from build123d import *


with BuildPart() as part:
    # Sweep1: sweep along a path in Sketch2
    with BuildLine(Plane(origin=(0, 0, 0), x_dir=(1, 0, 0), z_dir=(0, 1, 0))) as sweep1_path:
        Line((-1005, -399), (1005, -399))
        Line((1005, -399), (1005, 399))
        Line((1005, 399), (-1005, 399))
        Line((-1005, 399), (-1005, -399))
    # Sketch3 → Sweep1 (sweep)
    with BuildSketch(Plane.XY):
        Polygon((-955, 0), (-1005, 0), (-1005, 50), (-1000, 50), (-1000, 5), (-955, 5), align=None)
    sweep(path=sweep1_path.line, transition=Transition.RIGHT)


solid = part.part
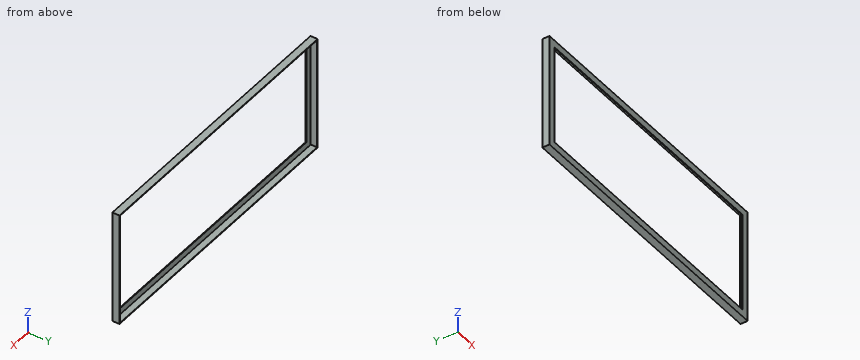
Design review of the part built by this model. Coordinates are the model's own, in mm. Coordinates: 2 decimals unless noted, no trailing zeros. Loops run counter-clockwise (first coordinate to the right, second up) from the corner with the lowest first, then second, coordinate; pieces in that order, holes last. Notation, with made-up numbers: M 12.5,38 L 48.5,38 A23 cw 48.5,72 Z; hole C 73,20 d4. An arc over 180 degrees is marked long. Use one line per item in the form item = value.
(1) Consider section C-C (y = 25). Write out the cut boundary in (x, z).
Return value:
outline = M -1005,-399 L 1005,-399 L 1005,399 L -1005,399 Z; hole M -1000,-394 L 1000,-394 L 1000,394 L -1000,394 Z
(2) Consider section A-A (x = -374). Write out the cut boundary in (y, z), and give its area (3 significant figures).
Return value:
outline = M 0,-399 L 50,-399 L 50,-394 L 5,-394 L 5,-349 L 0,-349 Z; M 0,349 L 5,349 L 5,394 L 50,394 L 50,399 L 0,399 Z
area = 950 mm2
(3) Consider section B-B (z = 168.5). Write out the cut boundary in (x, y), and give its area (3 significant figures).
Return value:
outline = M -1005,0 L -955,0 L -955,5 L -1000,5 L -1000,50 L -1005,50 Z; M 955,0 L 1005,0 L 1005,50 L 1000,50 L 1000,5 L 955,5 Z
area = 950 mm2
(4) For line 1 along Z through (x, y) = (69, 39.5); line 2 along X through (y, z) = (7.5, -339); line 3 along X through (y, z) = (4, -333), list the stretches that pass through material, from the lowest coordinate up. Write a range as from..to.
Return value:
line_1 = -399..-394, 394..399
line_2 = -1005..-1000, 1000..1005
line_3 = -1005..-955, 955..1005
